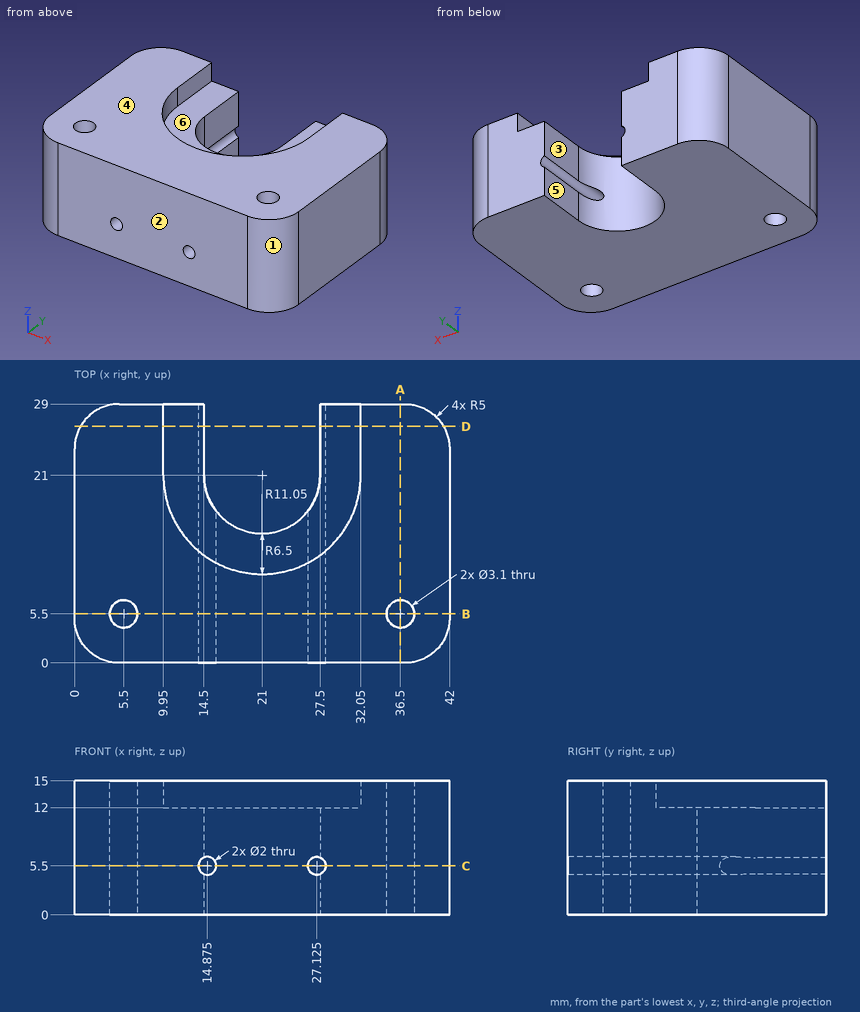
Input: dimensioned drawing with shaded views. Units: mm. Origin: part minimum x, y, z. A direction names the side the tool comes from. Round coordinates to 2 decimals unless told otherwise and drop trailing zeros. Loops run counter-clockwise (first coordinate to the right, second up) from the corner with the lowest first, then second, coordinate; pieces in that order, holes last. Notation, with made-up numbers: (40.25, 46) -> (79.25, 46) arc R28 cw to (79.25, 74) -> close; hole circle Ø8 at (88.25, 78.25). An arc over 180 degrees is marked (long way). Use one line per item in the form item = value. Start each with the question number.
1) Section D-D on y = 26.5. Output: boundary loops of the cut face in (x, z) (3 decimals), then the cut area to 3 significant figures.
2) Section C-C on z = 5.5. Output: boundary loops of the cut face in (x, y) (3 decimals).
3) First-contact query: P1, Ø2.5, axis at x = 5.5, y = 5.5, coming from the +Z side; P2, Ø0.9, axis at y = 25.5, z = 14, coming from the -X side; P3, Ø9.5, axis at x = 23, y = 16, coming from the +Z side; P4, Ø1.7, axis at y = 27, z = 8.5, coming from the -X side. Flat tips, straight axial feed; report the tip coordinate or a pass-through.
4) Section B-B on y = 5.5. Output: boundary loops of the cut face in (x, z) (3 decimals).
5) Draft query along X for the marked faces 1, 2 and 3. Return one class per face: released by +X, released by -X, zero draft, split by the parting line, or undercut.
6) Section A-A on x = 36.5. Output: boundary loops of the cut face in (y, z).
7) Line query: L1, parallel to X at y = 4.5, z = 9; L2, parallel to Y at x = 36.5, z = 5.5; L3, parallel to Z at x = 27, y = 4.25. Output: solid intervals per line, ascending.
8) Access query for the marked faces 4, 5 and 6. Directions: +Z, -Z, +X, -X, +Y, -Y. A direction counts if a zero-diameter tool reaches every point of the face in a straight line with its end or side. Return the directions, or none.
Response:
q1.outline = (0.67, 0) -> (14.5, 0) -> (14.5, 4.573) arc R1 cw to (14.5, 6.427) -> (14.5, 12) -> (9.95, 12) -> (9.95, 15) -> (0.67, 15) -> close; (27.5, 0) -> (41.33, 0) -> (41.33, 15) -> (32.05, 15) -> (32.05, 12) -> (27.5, 12) -> (27.5, 6.427) arc R1 cw to (27.5, 4.573) -> close
q1.area = 386 mm^2
q2.outline = (0, 5) arc R5 ccw to (5, 0) -> (13.875, 0) -> (13.875, 29) -> (5, 29) arc R5 ccw to (0, 24) -> close; (15.875, 0) -> (26.125, 0) -> (26.125, 17.002) arc R6.5 cw to (15.875, 17.002) -> close; (28.125, 0) -> (37, 0) arc R5 ccw to (42, 5) -> (42, 24) arc R5 ccw to (37, 29) -> (28.125, 29) -> close; hole circle Ø3.1 at (5.5, 5.5); hole circle Ø3.1 at (36.5, 5.5)
q3.P1 = through
q3.P2 = 0.11
q3.P3 = 12
q3.P4 = 0.49
q4.outline = (0, 0) -> (3.95, 0) -> (3.95, 15) -> (0, 15) -> close; (7.05, 0) -> (34.95, 0) -> (34.95, 15) -> (7.05, 15) -> close; (38.05, 0) -> (42, 0) -> (42, 15) -> (38.05, 15) -> close; hole circle Ø2 at (14.875, 5.5); hole circle Ø2 at (27.125, 5.5)
q5.face_1 = released by +X
q5.face_2 = zero draft
q5.face_3 = undercut
q6.outline = (0, 0) -> (3.95, 0) -> (3.95, 15) -> (0, 15) -> close; (7.05, 0) -> (29, 0) -> (29, 15) -> (7.05, 15) -> close
q7.L1 = 0.03 to 4.32, 6.68 to 35.32, 37.68 to 41.97
q7.L2 = 0 to 3.95, 7.05 to 29
q7.L3 = 0 to 4.51, 6.49 to 15
q8.face_4 = +Z, +X, -X, +Y, -Y
q8.face_5 = +Z, -Z, +Y
q8.face_6 = +Z, +Y
